Design review of the part built by this model. Coordinates are the model's own, in mm. A direction names the side the tool comes from. Coordinates: 2 decimals unless noted, no trailing zeros. Loops run counter-clockwise (first coordinate to the right, second up) from the corner with the lowest first, then second, coordinate; pieces in that order, holes last. Notation, with made-up numbers: M 44.5,28.25 L 72.5,28.25 A12 ccw 72.5,40.25 Z; hole C 52.5,-14.75 d2. An arc over 180 degrees is marked long. Put each result on its own line as item: value. Start each with the question number.
(1) For probe 1 along X at (y, z) = (2.25, 5); probe 2 along Z at (x, y) = (11, 2); probe 3 along Y at (x, z) = (9, 1.25), list the stretches that pass through material, from the lowest coordinate up. Write a range as [from, to].
(2) For faces 4 (the flat face through (2, 0, -3)), 5 (the flat face through (0, 2.5, 2.5)), list the 3-axis set-ups (+Z, -Z, +X, -X, +Y, -Y) from which the entire face can be reached by the end or side of a thin tool; tool diameter is ignored.
(3) Clearance check with flat-ended pins moving along their axes: pin 1 (6 mm diameter, centred on x = 28.5, z = -1, fed in from -Y); pin 2 (5 mm diameter, centred on x = 28.5, y = -4, fed in from +Z); pin 3 (4 mm diameter, centred on x = 9, y = 4, fed in from +Z). State where each tip first meets the part, or that it passes through.
(4) The part is to be moulded in two halves that separate along Z. For faces 1 (the flat face through (4, 1.5, -2.8)), 2 (the flat face through (38, 0, 0)), 3 (the cylindrical face through (4.45, 3.955, 5.158)), say which applies: +Z half, -Z half, draft (parallel to the pull), parting line (faces both ways), or undercut.
(5) Take a section at A-A, the plane x = 34. Give the boundary of the cut face in (y, z).
```python
from build123d import *

# Parameters (mm, degrees)
CHAMFER1_SIZE      = 0.625
CUT_EXTRUDE1_DEPTH = 4
CHAMFER2_SIZE      = 0.8
FILLET1_R          = 0.4


with BuildPart() as part:
    # Sketch1 → Revolve1 (revolve)
    with BuildSketch(Plane(origin=(0, 0, 0), x_dir=(1, 0, 0), z_dir=(0, 1, 0))):
        Polygon((0, 0), (0, 6.5), (8, 6.5), (8, 4), (38, 4), (38, 0), align=None)
    revolve(axis=Axis((38, 0, 0), (-1, 0, 0)))

    # Chamfer1
    chamfer1_edges = [part.edges().sort_by_distance(p)[0] for p in [
        (38, 0, 4),
    ]]
    chamfer(chamfer1_edges, length=CHAMFER1_SIZE)

    # Sketch3 → Cut-Revolve1 (revolve, cut)
    with BuildSketch(Plane(origin=(0, 0, 0), x_dir=(1, 0, 0), z_dir=(0, 1, 0)), mode=Mode.PRIVATE) as cut_revolve1_sk:
        Polygon((0, 0), (5.732050808, 0), (4, 3), (0, 3), align=None)
    revolve(cut_revolve1_sk.sketch.rotate(Axis((0, 0, 0), (1, 0, 0)), 180), axis=Axis((0, 0, 0), (1, 0, 0)), mode=Mode.SUBTRACT)

    # Sketch2 → Cut-Extrude1 (cut)
    with BuildSketch(Plane.ZY):
        Polygon((0, 3.464101615), (-3, 1.732050808), (-3, -1.732050808), (0, -3.464101615), (3, -1.732050808), (3, 1.732050808), align=None)
    extrude(amount=-CUT_EXTRUDE1_DEPTH, mode=Mode.SUBTRACT)

    # Chamfer2
    chamfer2_edges = [part.edges().sort_by_distance(p)[0] for p in [
        (0, 0, 6.5),
    ]]
    chamfer(chamfer2_edges, length=CHAMFER2_SIZE)

    # Fillet1
    fillet1_edges = [part.edges().sort_by_distance(p)[0] for p in [
        (8, 0, 4),
    ]]
    fillet(fillet1_edges, radius=FILLET1_R)


solid = part.part
```
Computed values:
1. probe 1: x = [0, 8]
1. probe 2: z = [-3.46, 3.46]
1. probe 3: y = [-3.8, 3.8]
2. face 4: -X
2. face 5: +Z, -Z, -X, +Y, -Y
3. pin 1: stops at y = -4
3. pin 2: stops at z = 3.71
3. pin 3: stops at z = 6.09
4. face 1: undercut
4. face 2: draft
4. face 3: parting line
5. outline: C 0,0 d8
